```python
from build123d import *

# Parameters (mm, degrees)
SKETCH_1_W          = 360
SKETCH_1_H          = 80
EXTRUDE_1_DEPTH     = 5
SKETCH_3_W          = 360
SKETCH_3_H          = 5
EXTRUDE_2_DEPTH     = 40
SKETCH_4_W          = 5
SKETCH_4_H          = 120
EXTRUDE_3_DEPTH     = 15
SKETCH_5_W          = 5
SKETCH_5_H          = 120
EXTRUDE_4_DEPTH     = 15
EXTRUDE_5_DEPTH     = 20
EXTRUDE_6_DEPTH     = 20
EXTRUDE_START       = -20
EXTRUDE_7_DEPTH     = 20
SKETCH_9_W          = 2
SKETCH_9_H          = 5
CUT_EXTRUDE_1_DEPTH = 100


with BuildPart() as part:
    # 草图1 → 凸台-拉伸1 (new body)
    with BuildSketch(Plane.XY):
        Rectangle(SKETCH_1_W, SKETCH_1_H)
    extrude(amount=EXTRUDE_1_DEPTH)

    # 草图3 → 凸台-拉伸2 (add)
    with BuildSketch(Plane.XZ.offset(40)):
        with Locations((0, 2.5)):
            Rectangle(SKETCH_3_W, SKETCH_3_H)
    extrude(amount=EXTRUDE_2_DEPTH)

    # 草图4 → 凸台-拉伸3 (add)
    with BuildSketch(Plane.ZY.offset(180)):
        with Locations((2.5, -20)):
            Rectangle(SKETCH_4_W, SKETCH_4_H)
    extrude(amount=EXTRUDE_3_DEPTH)

    # 草图5 → 凸台-拉伸4 (add)
    with BuildSketch(Plane(origin=(180, 0, 0), x_dir=(0, 0, -1), z_dir=(1, 0, 0))):
        with Locations((-2.5, -20)):
            Rectangle(SKETCH_5_W, SKETCH_5_H)
    extrude(amount=EXTRUDE_4_DEPTH)

    # 草图6 → 凸台-拉伸5 (add)
    with BuildSketch(Plane.XZ.offset(80)):
        Polygon((-195, 3.5), (-197, 4.654700538), (-197, 0.345299462), (-195, 1.5), align=None)
        Polygon((195, 1.5), (195, 3.5), (197, 4.654700538), (197, 0.345299462), align=None)
    extrude(amount=-EXTRUDE_5_DEPTH)

    # 草图7 → 凸台-拉伸6 (add)
    with BuildSketch(Plane(origin=(0, 40, 0), x_dir=(1, 0, 0), z_dir=(0, 1, 0))):
        Polygon((-195, -3.5), (-195, -1.5), (-197, -0.345299462), (-197, -4.654700538), align=None)
        Polygon((197, -0.345299462), (195, -1.5), (195, -3.5), (197, -4.654700538), align=None)
    extrude(amount=-EXTRUDE_6_DEPTH)

    # 草图8 → 凸台-拉伸7 (add)
    with BuildSketch(Plane(origin=(0, 0, 0), x_dir=(1, 0, 0), z_dir=(0, 1, 0)).offset(EXTRUDE_START)):
        Polygon((-195, -3.5), (-195, -1.5), (-197, -0.345299462), (-197, -4.654700538), align=None)
        Polygon((197, -0.345299462), (195, -1.5), (195, -3.5), (197, -4.654700538), align=None)
    extrude(amount=-EXTRUDE_7_DEPTH)

    # 草图9 → 切除-拉伸1 (cut)
    with BuildSketch(Plane.XZ.offset(80)):
        with Locations((10, 2.5)):
            Rectangle(SKETCH_9_W, SKETCH_9_H)
        with Locations((20, 2.5)):
            Rectangle(SKETCH_9_W, SKETCH_9_H)
        with Locations((0, 2.5)):
            Rectangle(SKETCH_9_W, SKETCH_9_H)
        with Locations((30, 2.5)):
            Rectangle(SKETCH_9_W, SKETCH_9_H)
        with Locations((40, 2.5)):
            Rectangle(SKETCH_9_W, SKETCH_9_H)
        with Locations((50, 2.5)):
            Rectangle(SKETCH_9_W, SKETCH_9_H)
        with Locations((60, 2.5)):
            Rectangle(SKETCH_9_W, SKETCH_9_H)
        with Locations((70, 2.5)):
            Rectangle(SKETCH_9_W, SKETCH_9_H)
        with Locations((80, 2.5)):
            Rectangle(SKETCH_9_W, SKETCH_9_H)
        with Locations((90, 2.5)):
            Rectangle(SKETCH_9_W, SKETCH_9_H)
        with Locations((100, 2.5)):
            Rectangle(SKETCH_9_W, SKETCH_9_H)
        with Locations((110, 2.5)):
            Rectangle(SKETCH_9_W, SKETCH_9_H)
        with Locations((120, 2.5)):
            Rectangle(SKETCH_9_W, SKETCH_9_H)
        with Locations((130, 2.5)):
            Rectangle(SKETCH_9_W, SKETCH_9_H)
        with Locations((140, 2.5)):
            Rectangle(SKETCH_9_W, SKETCH_9_H)
        with Locations((150, 2.5)):
            Rectangle(SKETCH_9_W, SKETCH_9_H)
        with Locations((160, 2.5)):
            Rectangle(SKETCH_9_W, SKETCH_9_H)
        with Locations((170, 2.5)):
            Rectangle(SKETCH_9_W, SKETCH_9_H)
        with Locations((180, 2.5)):
            Rectangle(SKETCH_9_W, SKETCH_9_H)
        with Locations((190, 2.5)):
            Rectangle(SKETCH_9_W, SKETCH_9_H)
        with Locations((-10, 2.5)):
            Rectangle(SKETCH_9_W, SKETCH_9_H)
        with Locations((-20, 2.5)):
            Rectangle(SKETCH_9_W, SKETCH_9_H)
        with Locations((-30, 2.5)):
            Rectangle(SKETCH_9_W, SKETCH_9_H)
        with Locations((-40, 2.5)):
            Rectangle(SKETCH_9_W, SKETCH_9_H)
        with Locations((-50, 2.5)):
            Rectangle(SKETCH_9_W, SKETCH_9_H)
        with Locations((-60, 2.5)):
            Rectangle(SKETCH_9_W, SKETCH_9_H)
        with Locations((-70, 2.5)):
            Rectangle(SKETCH_9_W, SKETCH_9_H)
        with Locations((-80, 2.5)):
            Rectangle(SKETCH_9_W, SKETCH_9_H)
        with Locations((-90, 2.5)):
            Rectangle(SKETCH_9_W, SKETCH_9_H)
        with Locations((-100, 2.5)):
            Rectangle(SKETCH_9_W, SKETCH_9_H)
        with Locations((-110, 2.5)):
            Rectangle(SKETCH_9_W, SKETCH_9_H)
        with Locations((-120, 2.5)):
            Rectangle(SKETCH_9_W, SKETCH_9_H)
        with Locations((-130, 2.5)):
            Rectangle(SKETCH_9_W, SKETCH_9_H)
        with Locations((-140, 2.5)):
            Rectangle(SKETCH_9_W, SKETCH_9_H)
        with Locations((-150, 2.5)):
            Rectangle(SKETCH_9_W, SKETCH_9_H)
        with Locations((-160, 2.5)):
            Rectangle(SKETCH_9_W, SKETCH_9_H)
        with Locations((-170, 2.5)):
            Rectangle(SKETCH_9_W, SKETCH_9_H)
        with Locations((-180, 2.5)):
            Rectangle(SKETCH_9_W, SKETCH_9_H)
        with Locations((-190, 2.5)):
            Rectangle(SKETCH_9_W, SKETCH_9_H)
    extrude(amount=-CUT_EXTRUDE_1_DEPTH, mode=Mode.SUBTRACT)


solid = part.part
```
Work out the finished part from the listing and answer in its coordinate system (mm). Give positions to 0.01 mm unless a question says otherwise; leave off trailing zeros. One line per item, written item: value. Start each with the question number.
1. Find the intervals of material crossed by probe 1 along X at (y, z) = (22.5, 3.8); probe 2 along Y at (x, z) = (-70.5, 2.65), in increasing order.
2. Each of these flat-tipped pins is pushed along its axis until it touches: P1, Ø1.6, axis at x = 50.5, z = 2, coming from the -Y side; P2, Ø1.5, axis at y = -49.5, z = 2, coming from the -X side; P3, Ø2.5, axis at y = -52.5, z = 2, coming from the +X side; P4, Ø1.6, axis at x = 30, z = 2, coming from the -Y side. Where does it stop, or does it pass through?
3. Find section A-A (y = -50). State how many separate pieces and enclosed holes the cut face has, and give its area (3 significant figures).
Reported:
1. probe 1: x = -197 to -195.52, -195 to 195, 195.52 to 197
1. probe 2: y = 20 to 40
2. P1: stops at y = -80
2. P2: stops at x = -195
2. P3: stops at x = 195
2. P4: stops at y = 20
3. separate pieces: 40
3. enclosed holes: 0
3. area: 1,560 mm²
